Study the drawing (mm; zero at the part's minimum x, y, z) and answer. Give positions to 0.01 mm unless a question says otherwise; leave off trailing zeros. Order: outer loops, then holes, each group sorted by start corner. A loop starts at its lowest first (then second) coordinate and runs counter-clockwise, first axis right, second up.
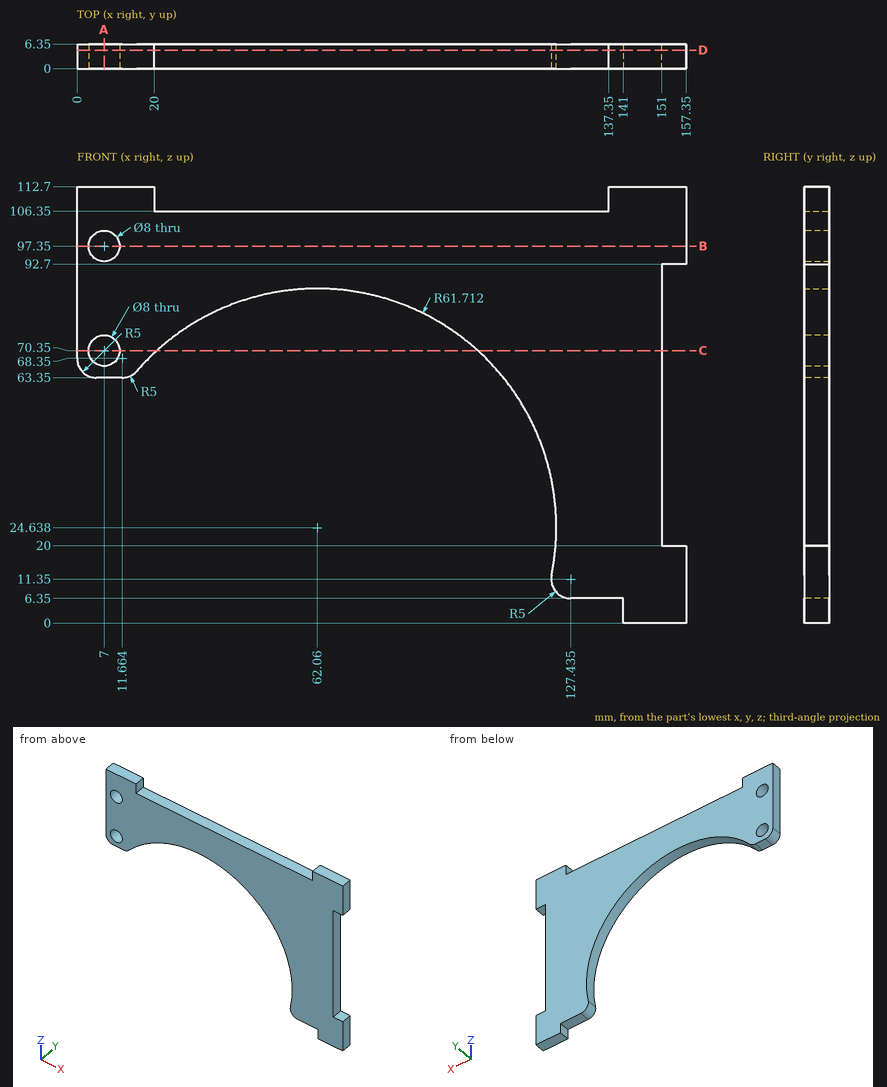
1) Find section B-B (z = 97.35). Write down the section's boundary in (x, y).
Geometry says:
outline: (0, 0) - (3, 0) - (3, 6.35) - (0, 6.35) - close; (11, 0) - (157.35, 0) - (157.35, 6.35) - (11, 6.35) - close
2) Find section C-C (z = 70.35). Write down the section's boundary in (x, y).
Geometry says:
outline: (0, 0) - (3, 0) - (3, 6.35) - (0, 6.35) - close; (11, 0) - (20.6, 0) - (20.6, 6.35) - (11, 6.35) - close; (103.52, 0) - (151, 0) - (151, 6.35) - (103.52, 6.35) - close
3) Find section D-D (y = 4.75). Count the separate pieces of the cut face and the enclosed holes in it, then the cut area to 3 significant figures.
Geometry says:
separate pieces: 1
enclosed holes: 2
area: 7,110 mm2
4) Find section A-A (x = 7). Write down the section's boundary in (y, z), then the cut area to 3 significant figures.
Geometry says:
outline: (0, 63.35) - (6.35, 63.35) - (6.35, 66.35) - (0, 66.35) - close; (0, 74.35) - (6.35, 74.35) - (6.35, 93.35) - (0, 93.35) - close; (0, 101.35) - (6.35, 101.35) - (6.35, 112.7) - (0, 112.7) - close
area: 212 mm2
5) Straight lines are drawn through the part: probe 1 along X at (y, z) = (4, 70.35); probe 2 along X at (y, z) = (2, 97.5); probe 3 along Z at (x, y) = (134.5, 1.5). For each, find the intervals that lie inside material, in ascending order.
Geometry says:
probe 1: x = 0 to 3, 11 to 20.6, 103.52 to 151
probe 2: x = 0 to 3, 11 to 157.35
probe 3: z = 6.35 to 106.35
6) Given P1, Ø1.9, axis at y = 2.5, z = 3, coming from the -X side; P2, Ø2, axis at y = 3, z = 58, coming from the +X side; P3, Ø1.9, axis at x = 8.5, y = 2.5, coming from the -Z side, each flat-ended and moving along its own axis, determine where each tip first touches the part or whether it passes through.
Geometry says:
P1: stops at x = 141
P2: stops at x = 151
P3: stops at z = 63.35
